```python
from build123d import *

# Parameters (mm, degrees)
SKETCH2_W           = 130
SKETCH2_H           = 90
BOSS_EXTRUDE1_DEPTH = 4
SKETCH3_R           = 1.5
CUT_EXTRUDE1_DEPTH  = 10
SKETCH4_R           = 1.6
CUT_EXTRUDE2_DEPTH  = 10
FILLET1_R           = 10
CUT_EXTRUDE3_DEPTH  = 10
SKETCH6_R           = 1.5
BOSS_EXTRUDE2_DEPTH = 4
SKETCH7_R           = 1.5
CUT_EXTRUDE4_DEPTH  = 10


with BuildPart() as part:
    # Sketch2 → Boss-Extrude1 (new body)
    with BuildSketch(Plane(origin=(0, 0, 0), x_dir=(1, 0, 0), z_dir=(0, 1, 0))):
        with Locations((71.271186441, 55.564971751)):
            Rectangle(SKETCH2_W, SKETCH2_H)
    extrude(amount=-BOSS_EXTRUDE1_DEPTH)

    # Sketch3 → Cut-Extrude1 (cut)
    with BuildSketch(Plane(origin=(0, 0, 0), x_dir=(1, 0, 0), z_dir=(0, 1, 0))):
        with Locations(Location((126.271186441, 63.564971751, 0), (0, 0, 270))):
            Circle(SKETCH3_R)
        with Locations(Location((126.271186441, 47.564971751, 0), (0, 0, 270))):
            Circle(SKETCH3_R)
        with Locations(Location((112.271186441, 47.564971751, 0), (0, 0, 270))):
            Circle(SKETCH3_R)
        with Locations(Location((112.271186441, 63.564971751, 0), (0, 0, 270))):
            Circle(SKETCH3_R)
        with Locations(Location((16.271186441, 47.564971751, 0), (0, 0, 90))):
            Circle(SKETCH3_R)
        with Locations(Location((30.271186441, 47.564971751, 0), (0, 0, 90))):
            Circle(SKETCH3_R)
        with Locations(Location((16.271186441, 63.564971751, 0), (0, 0, 90))):
            Circle(SKETCH3_R)
        with Locations(Location((30.271186441, 63.564971751, 0), (0, 0, 90))):
            Circle(SKETCH3_R)
    extrude(amount=-CUT_EXTRUDE1_DEPTH, mode=Mode.SUBTRACT)

    # Sketch4 → Cut-Extrude2 (cut)
    with BuildSketch(Plane(origin=(0, 0, 0), x_dir=(1, 0, 0), z_dir=(0, 1, 0))):
        with Locations(Location((16.271186441, 20.564971751, 0), (0, 0, 270))):
            Circle(SKETCH4_R)
        with Locations(Location((30.271186441, 20.564971751, 0), (0, 0, 270))):
            Circle(SKETCH4_R)
        with Locations(Location((30.271186441, 90.564971751, 0), (0, 0, 90))):
            Circle(SKETCH4_R)
        with Locations(Location((16.271186441, 90.564971751, 0), (0, 0, 90))):
            Circle(SKETCH4_R)
        with Locations(Location((112.271186441, 20.564971751, 0), (0, 0, 90))):
            Circle(SKETCH4_R)
        with Locations(Location((126.271186441, 20.564971751, 0), (0, 0, 90))):
            Circle(SKETCH4_R)
        with Locations(Location((126.271186441, 90.564971751, 0), (0, 0, 270))):
            Circle(SKETCH4_R)
        with Locations(Location((112.271186441, 90.564971751, 0), (0, 0, 270))):
            Circle(SKETCH4_R)
    extrude(amount=-CUT_EXTRUDE2_DEPTH, mode=Mode.SUBTRACT)

    # Fillet1
    fillet1_edges = [part.edges().sort_by_distance(p)[0] for p in [
        (6.271186441, -2, -100.564971751),
        (136.271186441, -2, -100.564971751),
        (136.271186441, -2, -10.564971751),
        (6.271186441, -2, -10.564971751),
    ]]
    fillet(fillet1_edges, radius=FILLET1_R)

    # Sketch5 → Cut-Extrude3 (cut)
    with BuildSketch(Plane(origin=(0, 0, 0), x_dir=(1, 0, 0), z_dir=(0, 1, 0))):
        with BuildLine():
            Line((76.271186441, 89.564971751), (76.271186441, 64.564971751))
            ThreePointArc((76.271186441, 64.564971751), (77.442759316, 61.736544627), (80.271186441, 60.564971751))
            Line((80.271186441, 60.564971751), (98.271186441, 60.564971751))
            ThreePointArc((98.271186441, 60.564971751), (101.099613565, 61.736544627), (102.271186441, 64.564971751))
            Line((102.271186441, 64.564971751), (102.271186441, 89.564971751))
            ThreePointArc((102.271186441, 89.564971751), (101.099613565, 92.393398876), (98.271186441, 93.564971751))
            Line((98.271186441, 93.564971751), (80.271186441, 93.564971751))
            ThreePointArc((80.271186441, 93.564971751), (77.442759316, 92.393398876), (76.271186441, 89.564971751))
        make_face()
        with BuildLine():
            Line((40.271186441, 89.564971751), (40.271186441, 64.564971751))
            ThreePointArc((40.271186441, 64.564971751), (41.442759316, 61.736544627), (44.271186441, 60.564971751))
            Line((44.271186441, 60.564971751), (62.271186441, 60.564971751))
            ThreePointArc((62.271186441, 60.564971751), (65.099613565, 61.736544627), (66.271186441, 64.564971751))
            Line((66.271186441, 64.564971751), (66.271186441, 89.564971751))
            ThreePointArc((66.271186441, 89.564971751), (65.099613565, 92.393398876), (62.271186441, 93.564971751))
            Line((62.271186441, 93.564971751), (44.271186441, 93.564971751))
            ThreePointArc((44.271186441, 93.564971751), (41.442759316, 92.393398876), (40.271186441, 89.564971751))
        make_face()
        with BuildLine():
            Line((66.271186441, 21.564971751), (66.271186441, 46.564971751))
            ThreePointArc((66.271186441, 46.564971751), (65.099613565, 49.393398876), (62.271186441, 50.564971751))
            Line((62.271186441, 50.564971751), (44.271186441, 50.564971751))
            ThreePointArc((44.271186441, 50.564971751), (41.442759316, 49.393398876), (40.271186441, 46.564971751))
            Line((40.271186441, 46.564971751), (40.271186441, 21.564971751))
            ThreePointArc((40.271186441, 21.564971751), (41.442759316, 18.736544627), (44.271186441, 17.564971751))
            Line((44.271186441, 17.564971751), (62.271186441, 17.564971751))
            ThreePointArc((62.271186441, 17.564971751), (65.099613565, 18.736544627), (66.271186441, 21.564971751))
        make_face()
        with BuildLine():
            Line((102.271186441, 21.564971751), (102.271186441, 46.564971751))
            ThreePointArc((102.271186441, 46.564971751), (101.099613565, 49.393398876), (98.271186441, 50.564971751))
            Line((98.271186441, 50.564971751), (80.271186441, 50.564971751))
            ThreePointArc((80.271186441, 50.564971751), (77.442759316, 49.393398876), (76.271186441, 46.564971751))
            Line((76.271186441, 46.564971751), (76.271186441, 21.564971751))
            ThreePointArc((76.271186441, 21.564971751), (77.442759316, 18.736544627), (80.271186441, 17.564971751))
            Line((80.271186441, 17.564971751), (98.271186441, 17.564971751))
            ThreePointArc((98.271186441, 17.564971751), (101.099613565, 18.736544627), (102.271186441, 21.564971751))
        make_face()
    extrude(amount=-CUT_EXTRUDE3_DEPTH, mode=Mode.SUBTRACT)

    # Sketch6 → Boss-Extrude2 (add)
    with BuildSketch(Plane(origin=(0, 0, 0), x_dir=(1, 0, 0), z_dir=(0, 1, 0))):
        with Locations((30.271186441, 63.564971751)):
            Circle(SKETCH6_R)
        with Locations((30.271186441, 47.564971751)):
            Circle(SKETCH6_R)
        with Locations((16.271186441, 47.564971751)):
            Circle(SKETCH6_R)
        with Locations((16.271186441, 63.564971751)):
            Circle(SKETCH6_R)
        with Locations((112.271186441, 63.564971751)):
            Circle(SKETCH6_R)
        with Locations((126.271186441, 63.564971751)):
            Circle(SKETCH6_R)
        with Locations((126.271186441, 47.564971751)):
            Circle(SKETCH6_R)
        with Locations((112.271186441, 47.564971751)):
            Circle(SKETCH6_R)
    extrude(amount=-BOSS_EXTRUDE2_DEPTH)

    # Sketch7 → Cut-Extrude4 (cut)
    with BuildSketch(Plane(origin=(0, 0, 0), x_dir=(1, 0, 0), z_dir=(0, 1, 0))):
        with Locations(Location((71.271186441, 75.814971751, 0), (0, 0, 270))):
            Circle(SKETCH7_R)
        with Locations(Location((71.271186441, 33.814971751, 0), (0, 0, 270))):
            Circle(SKETCH7_R)
    extrude(amount=-CUT_EXTRUDE4_DEPTH, mode=Mode.SUBTRACT)


solid = part.part
```
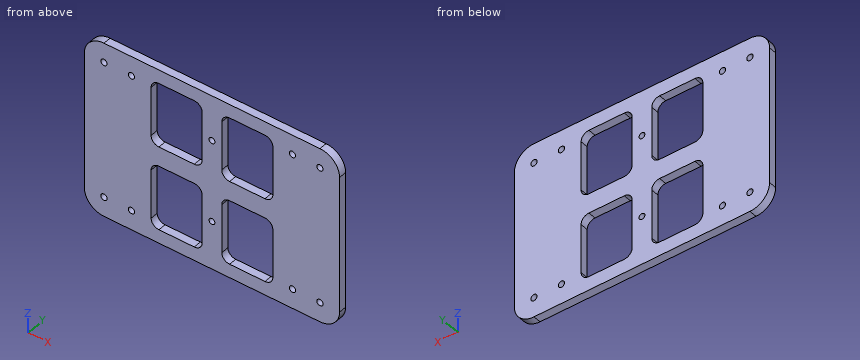
Check sheet for the modelled part. Datum: model origin and axes. Units: mm. Give positions to 0.01 mm unless a question says otherwise; leave off trailing zeros. Order: outer loops, then holes, each group sorted by start corner. A loop starts at its lowest first (then second) coordinate and runs counter-clockwise, first axis right, second up. Notation, with made-up numbers: M 37,39.5 L 93,39.5 A17 ccw 93,48.5 Z; hole C 70.25,-8.75 d2. An arc over 180 degrees is marked long. Answer in a Markdown table with one row per item. Add a question column.
Q1. Thickness scan on L1, parallel to X at y = -3.2, z = -87; L2, parallel to Z at x = 49.5, y = -3.8; L3, parallel to X at y = -1.25, z = -62. Record the ranges inside material, lowest first.
Q2. Sectioned sample at C-C, the plane y = -2.25. Count the separate pieces of the cut face and the enclosed holes in it, and give its area (3 significant figures).
Q3. Sectioned sample at B-B, the plane x = 58. Record the boundary of the cut face in (y, z), and give its area (3 significant figures).
Q4. Sectioned sample at A-A, the plane z = -69. Record the boundary of the cut face in (x, y), and give its area (3 significant figures).
Verdict:
| question | item | result |
|---|---|---|
| 1 | L1 | 6.27 to 40.27, 66.27 to 76.27, 102.27 to 136.27 |
| 1 | L2 | -100.56 to -93.56, -60.56 to -50.56, -17.56 to -10.56 |
| 1 | L3 | 6.27 to 41.2, 65.34 to 77.2, 101.34 to 136.27 |
| 2 | separate pieces | 1 |
| 2 | enclosed holes | 14 |
| 2 | area | 8,160 mm² |
| 3 | outline | M -4,-100.56 L 0,-100.56 L 0,-93.56 L -4,-93.56 Z; M -4,-60.56 L 0,-60.56 L 0,-50.56 L -4,-50.56 Z; M -4,-17.56 L 0,-17.56 L 0,-10.56 L -4,-10.56 Z |
| 3 | area | 96.0 mm² |
| 4 | outline | M 6.27,-4 L 40.27,-4 L 40.27,0 L 6.27,0 Z; M 66.27,-4 L 76.27,-4 L 76.27,0 L 66.27,0 Z; M 102.27,-4 L 136.27,-4 L 136.27,0 L 102.27,0 Z |
| 4 | area | 312 mm² |
